Input: part model. Units: mm. Frame: model coordinates. Coordinates: 2 decimals unless noted, no trailing zeros. Loops run counter-clockwise (first coordinate to the right, second up) from the corner with the lowest first, then second, coordinate; pieces in that order, holes last. Notation, with made-up numbers: (50.25, 6.25) - (90.25, 6.25) arc R12 cw to (90.25, 14.25) - close; hole circle Ø9 at (28.5, 11.25). An arc over 180 degrees is marked (long way). Write item = value, one per line. Start each with the question number.
from build123d import *

# Parameters (mm, degrees)
BOSS_EXTRUDE1_DEPTH = 0.635
CHAMFER1_SIZE       = 0.2


with BuildPart() as part:
    # Sketch1 → Boss-Extrude1 (new body)
    with BuildSketch(Plane(origin=(0, 0, 0), x_dir=(0, 0, -1), z_dir=(1, 0, 0))):
        with BuildLine():
            Line((0.635, 1.5), (0.635, 10.2175))
            Line((0.635, 10.2175), (0, 10.2175))
            Line((0, 10.2175), (0, 1.5))
            ThreePointArc((0, 1.5), (0.439339828, 0.439339828), (1.5, 0))
            Line((1.5, 0), (4.887, 0))
            Line((4.887, 0), (4.887, 0.635))
            Line((4.887, 0.635), (1.5, 0.635))
            ThreePointArc((1.5, 0.635), (0.888352634, 0.888352634), (0.635, 1.5))
        make_face()
    extrude(amount=-BOSS_EXTRUDE1_DEPTH)

    # Chamfer1
    chamfer1_edges = [part.edges().sort_by_distance(p)[0] for p in [
        (-0.635, 0.3175, -4.887),
        (-0.3175, 10.2175, 0),
        (-0.3175, 10.2175, -0.635),
        (-0.3175, 0.635, -4.887),
        (-0.3175, 0, -4.887),
        (-0.635, 10.2175, -0.3175),
        (0, 10.2175, -0.3175),
        (0, 0.3175, -4.887),
    ]]
    chamfer(chamfer1_edges, length=CHAMFER1_SIZE)


solid = part.part
Item 1: Pin query (flat end, axial travel): pin 1 (1 mm diameter, centred on y = 6, z = -2, fed in from -X). Return the tip coordinate at first contact, or that it passes through.
Item 2: Cut plane C-C on z = -2. Return loops of the section in (x, y) (3 decimals), plus the area to 3 significant figures.
Item 3: Ray query, line 1 (Z direction, x = -0.25, y = 2) (3 decimals); line 2 (Y direction, x = -0.15, z = -2) (3 decimals); line 3 (Y direction, x = -0.6, z = -0.45). Return the intervals inside material, ascending.
Item 4: Cut plane B-B on y = 4. Return loops of the section in (x, z) (3 decimals).
Recorded:
q1.pin_1 = through
q2.outline = (-0.635, 0) - (0, 0) - (0, 0.635) - (-0.635, 0.635) - close
q2.area = 0.403 mm²
q3.line_1 = -0.635 to 0
q3.line_2 = 0 to 0.635
q3.line_3 = 0.43 to 10.05
q4.outline = (-0.635, -0.635) - (0, -0.635) - (0, 0) - (-0.635, 0) - close
